```python
from build123d import *

# Parameters (mm, degrees)
SKETCH4_R           = 28.575
BOSS_EXTRUDE2_DEPTH = 0.254
SKETCH5_R           = 15.875
CUT_EXTRUDE5_DEPTH  = 1.254
SKETCH6_R           = 4.699
CUT_EXTRUDE6_DEPTH  = 1.254
SKETCH8_OUTSIDE_W   = 75.314
SKETCH8_OUTSIDE_H   = 75.314
CUT_EXTRUDE11_DEPTH = 1.254


with BuildPart() as part:
    # Sketch4 → Boss-Extrude2 (new body)
    with BuildSketch(Plane.XY):
        Circle(SKETCH4_R)
    extrude(amount=BOSS_EXTRUDE2_DEPTH)

    # Sketch5 → Cut-Extrude5 (cut, through all)
    with BuildSketch(Plane.XY.offset(0.254)):
        Circle(SKETCH5_R)
    extrude(amount=-CUT_EXTRUDE5_DEPTH, mode=Mode.SUBTRACT)

    # Sketch6 → Cut-Extrude6 (cut, through all)
    with BuildSketch(Plane.XY.offset(0.254)):
        with Locations((22.225, 0)):
            Circle(SKETCH6_R)
    extrude(amount=-CUT_EXTRUDE6_DEPTH, mode=Mode.SUBTRACT)

    # Sketch8 outside → Cut-Extrude11 (cut, through all)
    with BuildSketch(Plane.XY.offset(0.254)):
        Rectangle(SKETCH8_OUTSIDE_W, SKETCH8_OUTSIDE_H)
        with BuildLine():
            Line((15.105587123, 4.88230096), (26.859778778, 9.751046558))
            ThreePointArc((26.859778778, 9.751046558), (28.575, 0), (26.859778778, -9.751046558))
            Line((26.859778778, -9.751046558), (15.105587123, -4.88230096))
            ThreePointArc((15.105587123, -4.88230096), (15.875, 0), (15.105587123, 4.88230096))
        make_face(mode=Mode.SUBTRACT)
    extrude(amount=-CUT_EXTRUDE11_DEPTH, mode=Mode.SUBTRACT)


solid = part.part
```
Geometry check sheet. Reference: the model listing, model coordinates, mm. Coordinates: 2 decimals unless noted, no trailing zeros. Write each loop counter-clockwise with the first axis right and the second up, starting at its lowest first coordinate (ties: lowest second). Pieces come first, ordered by that corner, then holes. Notation, with made-up numbers: M 18,-31.75 L 73,-31.75 A21 cw 73,-22.75 Z; hole C -35.75,83 d7. An arc over 180 degrees is marked long. Answer as a JSON object with one key per item and string values.
1. Section check A-A, the plane y = 0. Enter the section's corners in (x, z) (3 decimals), plus the area to 3 significant figures.
Answers below:
{"outline": "M 15.875,0 L 17.526,0 L 17.526,0.254 L 15.875,0.254 Z; M 26.924,0 L 28.575,0 L 28.575,0.254 L 26.924,0.254 Z", "area": "0.839 mm²"}
2. Scan lines: L1, parallel to X at y = 1, z = 0.2; L2, parallel to Y at x = 22.5, z = 0.05; L3, parallel to Y at x = 26, z = 0.1. Record each from-to range of solid material in increasing order.
Answers below:
{"L1": "x = 15.84 to 17.63, 26.82 to 28.56", "L2": "y = -7.95 to -4.69, 4.69 to 7.95", "L3": "y = -9.39 to -2.8, 2.8 to 9.39"}
3. Section check D-D, the plane x = 16.5. Enter the section's corners in (y, z), plus the area to 3 significant figures.
Answers below:
{"outline": "M -5.46,0 L 5.46,0 L 5.46,0.25 L -5.46,0.25 Z", "area": "2.77 mm²"}
4. Section check B-B, the plane z = 0.05. Enter the section's corners in (x, y) (3 decimals).
Answers below:
{"outline": "M 15.106,-4.882 L 26.86,-9.751 A28.575 ccw 26.86,9.751 L 15.106,4.882 A15.875 cw Z; hole C 22.225,0 d9.398"}
5. Section check C-C, the plane y = 3.25. Enter the section's corners in (x, z).
Answers below:
{"outline": "M 15.54,0 L 18.83,0 L 18.83,0.25 L 15.54,0.25 Z; M 25.62,0 L 28.39,0 L 28.39,0.25 L 25.62,0.25 Z"}
6. Go/stop test with a flat-tipped pin: pin 1 Ø1 at (x, y) = (18.5, 4.5) entering from -Z. Record where the tip stops, or that it passes through.
Answers below:
{"pin 1": "stops at z = 0"}
